Check sheet for the modelled part. Datum: model origin and axes. Units: mm. A direction names the side the tool comes from. Coordinates: 2 decimals unless noted, no trailing zeros. Loops run counter-clockwise (first coordinate to the right, second up) from the corner with the lowest first, then second, coordinate; pieces in that order, holes last. Notation, with made-up numbers: M 37,-26 L 52,-26 A33 ccw 52,3 Z; hole C 53,65.25 d4. An arc over 180 degrees is marked long. Answer in a Markdown table with one row per item. Add a question column.
Autodesk Inventor part; units mm, degrees
ref_plane "YZ Plane" through (0, 0, 0) normal (1, 0, 0) x (0, 1, 0)
ref_plane "XZ Plane" through (0, 0, 0) normal (0, 1, 0) x (-1, 0, 0)
ref_plane "XY Plane" through (0, 0, 0) normal (0, 0, 1) x (1, 0, 0)
sketch "Skizze1" plane through (0, 0, 0) normal (0, 1, 0) x (-1, 0, 0)
  line L0 (115, 115) -> (-115, 115)
  line L1 (-115, 115) -> (-115, -115)
  line L2 (-115, -115) -> (115, -115)
  line L3 (115, -115) -> (115, 115)
  point P0 (0, 0)
  dimension "d0" = 230
  dimension "d1" = 230
extrude "Extrusion1" add sketch "Skizze1" along normal blind 1000
sketch "Skizze2" plane through (115, 0, 115) normal (1, 0, 0) x (0, 0, -1)
  line L0 (0, 0) -> (230, 0)
  line L1 (10, 0) -> (220, 0)
  line L2 (220, 0) -> (220, 180)
  line L3 (220, 180) -> (10, 180)
  line L4 (10, 180) -> (10, 0)
  point P0 (115, 0)
  dimension "d4" = 210
  dimension "d5" = 180
extrude "Extrusion2" cut sketch "Skizze2" against normal blind 230
sketch "Skizze3" plane through (0, 1000, 0) normal (0, 1, 0) x (1, 0, 0)
  circle A0 centre (0, 0) radius 105
  dimension "d8" = 210
extrude "Extrusion3" cut sketch "Skizze3" against normal blind 820
chamfer "Fase1" distance 2 angle 45 1 edges at (-105, 1000, 0)
sketch "Skizze4" plane through (115, 0, -115) normal (0, 0, -1) x (-1, 0, 0)
  line L0 (230, 0) -> (0, 0)
  line L1 (230, 180) -> (230, 0)
  line L2 (0, 0) -> (230, 0)
  line L3 (230, 0) -> (230, 10)
  line L4 (230, 10) -> (0, 10)
  line L5 (0, 10) -> (0, 0)
  point P0 (115, 0)
  dimension "d14" = 10
extrude "Extrusion4" add sketch "Skizze4" along normal blind 40
sketch "Skizze5" plane through (-115, 0, 115) normal (0, 0, 1) x (1, 0, 0)
  line L0 (230, 0) -> (0, 0)
  line L1 (230, 180) -> (230, 0)
  line L2 (0, 0) -> (230, 0)
  line L3 (230, 0) -> (230, 10)
  line L4 (230, 10) -> (0, 10)
  line L5 (0, 10) -> (0, 0)
  point P0 (115, 0)
  dimension "d17" = 10
extrude "Extrusion5" add sketch "Skizze5" along normal blind 40
sketch "Skizze6" plane through (-115, 10, 115) normal (0, 1, 0) x (1, 0, 0)
  line L0 (230, -40) -> (0, -40)
  line L1 (0, -40) -> (20, -40)
  line L2 (20, -40) -> (20, -20)
  line L3 (20, -20) -> (0, -20)
  line L4 (0, -20) -> (0, -40)
  line L5 (230, 0) -> (230, -40)
  line L6 (230, -40) -> (210, -40)
  line L7 (210, -40) -> (210, -20)
  line L8 (210, -20) -> (230, -20)
  line L9 (230, -20) -> (230, -40)
  line L10 (230, 270.1888) -> (210, 270.1888)
  line L11 (210, 270.1888) -> (210, 250.1888)
  line L12 (210, 250.1888) -> (230, 250.1888)
  line L13 (230, 250.1888) -> (230, 270.1888)
  line L14 (0, 270) -> (230, 270)
  line L15 (0, 270) -> (20, 270)
  line L16 (20, 270) -> (20, 250)
  line L17 (20, 250) -> (0, 250)
  line L18 (0, 250) -> (0, 270)
  point P0 (115, 115)
  dimension "d20" = 20
  dimension "d21" = 20
  dimension "d22" = 20
  dimension "d23" = 20
  dimension "d24" = 20
hole "Bohrung1" at (-95, 10, 135) at (95, 10, 135) at (-95, 10, -135) at (95, 10, -135.1888) direction (0, -1, 0) diameter 10 depth 10 tip angle 118 countersink diameter 14 countersink angle 90
properties part number "Magazin"
Q1. Cross-section at A-A (z = 0). Record the cut outline in (x, y), plus the area to 3 significant figures.
Q2. Thickness scan on L1, parallel to Z at x = 95, y = 5.5; L2, parallel to X at y = 4.75, z = 135; L3, parallel to Z at x = -95, y = 5. Record the ranges inside material, lowest first.
Q3. Mould release check, pull along X, two halves, no side actions. Record for faces 6 (the face through (2, 89, -105)), 7 (the face through (115, 618, -2)), 8 (the face through (-22.79, 998.13, 102.63)), 9 (the face through (-115, 618, -2)): released by +X, released by -X, zero draft, split by the parting line, or undercut.
Q4. Access from +Z, -Z, +X, -X, +Y, -Y to the whole of each face (thin tool, end or side, straight path). Record for faces 1 (the face through (109, 180, 0)), 2 (the face through (94, 1000, 52)), 3 (the face through (-2, 10, -135)), 4 (the face through (2, 10, 135)), 5 (the face through (100.15, 594.73, -31.54)).
Q5. Cross-section at B-B (y = 505). Record the cut outline in (x, z).
Q6. Go/stop test with flat-tipped pins: pin 1 (12 mm diameter, centred on x = 34.5, z = 125, fed in from +Y); pin 2 (3 mm diameter, centred on x = 82.5, y = 261.5, fed in from -Z). Record where each tip stops, or that it passes through.
Answer key:
| question | item | result |
|---|---|---|
| 1 | outline | M -115,180 L -105,180 L -105,998 L -107,1000 L -115,1000 Z; M 105,180 L 115,180 L 115,1000 L 107,1000 L 105,998 Z |
| 1 | area | 16,400 mm^2 |
| 2 | L1 | -155 to -140.19, -130.19 to -105, 105 to 130, 140 to 155 |
| 2 | L2 | -115 to -100, -90 to 90, 100 to 115 |
| 2 | L3 | -155 to -140, -130 to -105, 105 to 130, 140 to 155 |
| 3 | face 6 | zero draft |
| 3 | face 7 | released by +X |
| 3 | face 8 | undercut |
| 3 | face 9 | released by -X |
| 4 | face 1 | +X, -X, -Y |
| 4 | face 2 | +Z, -Z, +X, -X, +Y |
| 4 | face 3 | -Z, +X, -X, +Y |
| 4 | face 4 | +Z, +X, -X, +Y |
| 4 | face 5 | +Y, -Y |
| 5 | outline | M -115,-115 L 115,-115 L 115,115 L -115,115 Z; hole C 0,0 d210 |
| 6 | pin 1 | y = 10 |
| 6 | pin 2 | z = -115 |
